Read the model definition and answer for the solid it produces. Units are mm, in the model's axes. A direction names the side the tool comes from. Coordinates: 2 decimals unless noted, no trailing zeros. Loops run counter-clockwise (first coordinate to the right, second up) from the corner with the lowest first, then second, coordinate; pieces in that order, holes last. Notation, with made-up numbers: (61.5, 31) -> (89.5, 31) arc R20 ccw to (89.5, 53) -> close; hole circle Ø8 at (-14, 35.25). An arc over 180 degrees is marked (long way). Answer as a JSON object with one key per item and string values. Group by question number.
Q1. The part is cut by section C-C on z = 43.5. Write down the section's boundary in (x, y).
Q2. For faces 1 (the cylindrical face through (44.675, -42.737, 68.717)), 2 (the flat face through (50.8, -26, 38)), 3 (the flat face through (25, -12.7, 39)), determine the directions among +Z, -Z, +X, -X, +Y, -Y from which every point of the face is accessible in a straight line to the end or side of a thin tool.
Q3. The part is cut by section B-B on y = -24. Write down the section's boundary in (x, z), and give its area (3 significant figures).
Q4. The part is cut by section A-A on z = 66.5. Write down the section's boundary in (x, y).
Q5. Each of these flat-tipped pins is pushed along its axis until it touches: P1, Ø4.5, axis at x = 6.35, y = -44.45, coming from the +Z side; P2, Ø8, axis at x = 29.5, y = -17.5, coming from the -Z side; P3, Ø3, axis at x = 6.35, y = -6.35, coming from the +Z side. Where does it stop, or does it pass through?
Q6. Determine the mould class of faces 4 (the flat face through (25, -50.8, 38)), 5 (the flat face through (38.1, -26, 39)), 6 (the flat face through (25, -8, 0)) for opening direction Y: released by +Y, released by -Y, zero draft, split by the parting line, or undercut.
Q7. Straight lines are drawn through the part: line 1 along Y through (x, z) = (6.35, 71); line 2 along X through (y, z) = (-44.45, 70.75); line 3 along Y through (x, z) = (34.5, 54.5). For each, find the intervals that lie inside material, in ascending order. Write a range as [from, to].
from build123d import *

# Parameters (mm, degrees)
F0_W           = 50.8
F0_H           = 50.8
F1_DEPTH       = 76.2
F2_W           = 25.4
F2_H           = 25.4
F3_DEPTH       = 76.201
F5_D           = 3.4544
F5_DEPTH       = 12.7
F5_CSINK_D     = 7.1374
F5_CSINK_ANGLE = 82
F5_TIP         = 1.0378064612


with BuildPart() as f1:
    # F0 (on Top) → F1 (new body)
    with BuildSketch(Plane.XY):
        with Locations((25.4, -25.4)):
            Rectangle(F0_W, F0_H)
    extrude(amount=F1_DEPTH)

    # F2 (on face) → F3 (cut, through all)
    with BuildSketch(Plane.XY.offset(76.2)):
        with Locations((25.4, -25.4)):
            Rectangle(F2_W, F2_H)
    extrude(amount=-F3_DEPTH, mode=Mode.SUBTRACT)

    # F5
    with Locations(Plane.XY.offset(76.2)):
        with Locations((6.35, -6.35), (44.45, -6.35), (44.45, -44.45), (6.35, -44.45)):
            CounterSinkHole(F5_D / 2, F5_CSINK_D / 2, depth=F5_DEPTH, counter_sink_angle=F5_CSINK_ANGLE)
            with Locations((0, 0, -(F5_DEPTH + F5_TIP / 2))):  # 118° drill point
                Cone(0, F5_D / 2, F5_TIP, mode=Mode.SUBTRACT)


solid = f1.part
Final values:
{
 "1": {"outline": "(0, -50.8) -> (50.8, -50.8) -> (50.8, 0) -> (0, 0) -> close; hole (12.7, -38.1) -> (38.1, -38.1) -> (38.1, -12.7) -> (12.7, -12.7) -> close"},
 "2": {"face 1": "+Z", "face 2": "+Z, -Z, +X, +Y, -Y", "face 3": "+Z, -Z"},
 "3": {"outline": "(0, 0) -> (12.7, 0) -> (12.7, 76.2) -> (0, 76.2) -> close; (38.1, 0) -> (50.8, 0) -> (50.8, 76.2) -> (38.1, 76.2) -> close", "area": "1,940 mm2"},
 "4": {"outline": "(0, -50.8) -> (50.8, -50.8) -> (50.8, 0) -> (0, 0) -> close; hole circle Ø3.45 at (6.35, -44.45); hole circle Ø3.45 at (6.35, -6.35); hole (12.7, -38.1) -> (38.1, -38.1) -> (38.1, -12.7) -> (12.7, -12.7) -> close; hole circle Ø3.45 at (44.45, -44.45); hole circle Ø3.45 at (44.45, -6.35)"},
 "5": {"P1": "stops at z = 74.68", "P2": "passes through", "P3": "stops at z = 63.36"},
 "6": {"face 4": "released by -Y", "face 5": "undercut", "face 6": "zero draft"},
 "7": {"line 1": "y = [-50.8, -46.18], [-42.72, -8.08], [-4.62, 0]", "line 2": "x = [0, 4.62], [8.08, 42.72], [46.18, 50.8]", "line 3": "y = [-50.8, -38.1], [-12.7, 0]"}
}
